Design review of the part built by this model. Coordinates are the model's own, in mm. Face numbers are marked on the shaded views. A direction names the side the tool comes from. Give positions to 0.01 mm unless a question says otherwise; leave off trailing zeros. Order: outer loops, then holes, each group sorted by start corner. A loop starts at its lowest first (then second) coordinate and runs counter-clockwise, first axis right, second up. Notation, with made-up numbers: (83, -39) -> (110, -39) arc R23 ccw to (110, -27) -> close; hole circle Ø9 at (43.25, 81). An arc over 180 degrees is marked (long way). Return JSON: item names as keys, results as strings.
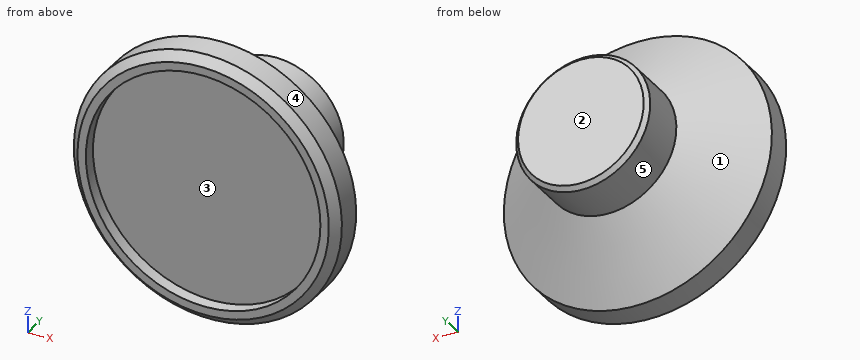
```python
from build123d import *

# Parameters (mm, degrees)
F2_SIZE  = 0.79375
F3_SIZE  = 1.5875
F4_R     = 22.225
F5_DEPTH = 2.3622


with BuildPart() as f1:
    # F0 (on Right) → F1 (revolve)
    with BuildSketch(Plane.YZ):
        Polygon((0, 25.4), (0, 0), (25.4, 0), (25.4, 12.7), (15.875, 12.7), (6.35, 25.4), align=None)
    revolve(axis=Axis((0, 12.7, 0), (0, -1, 0)))

    # F2
    f2_edges = [f1.edges().sort_by_distance(p)[0] for p in [
        (0, 25.4, -12.7),
    ]]
    chamfer(f2_edges, length=F2_SIZE)

    # F3
    f3_edges = [f1.edges().sort_by_distance(p)[0] for p in [
        (0, 0, -25.4),
    ]]
    chamfer(f3_edges, length=F3_SIZE)

    # F4 (on face) → F5 (cut)
    with BuildSketch(Plane.XZ):
        Circle(F4_R)
    extrude(amount=-F5_DEPTH, mode=Mode.SUBTRACT)


solid = f1.part
```
Item 1: Machinability: for the marked faces 4 and 5, which of the approach directions +Z, -Z, +X, -X, +Y, -Y give a long, thin tool a straight path to every point of the face, cutting with its end or side? Answer none if there is none.
Result set:
{"face 4": "+Y, -Y", "face 5": "+Y"}
Item 2: Wall thickness on L1, parallel to Z at x = 0, y = 0.5 (1 decimal); L2, parallel to Z at x = 0, y = 0.65 (1 decimal); L3, parallel to Y at x = -6.5, z = -8: over which ranges is each line inside the solid? List them lowest first. Write a range as [from, to].
Result set:
{"L1": "z = [-24.3, -22.2], [22.2, 24.3]", "L2": "z = [-24.5, -22.2], [22.2, 24.5]", "L3": "y = [2.36, 25.4]"}
Item 3: Add section C-C (y = 11.25). Give the boundary of the cut face in (x, z).
Result set:
{"outline": "circle Ø37.73 at (0, 0)"}
Item 4: Mouldability with a two-part tool opening along Z and no side actions: class the marked faces 1, 2 and 3 as released by +Z, released by -Z, zero draft, split by the parting line, or undercut.
Result set:
{"face 1": "split by the parting line", "face 2": "zero draft", "face 3": "undercut"}
Item 5: For pin 1 (3 mm diameter, centred on x = -12.5, z = -20, fed in from +Y); pin 2 (4 mm diameter, centred on x = -7, z = -13, fed in from -Y); pin 3 (6 mm diameter, centred on x = -18, y = 4.5, fed in from +Z), all flat-tipped, find the tip position at first contact; note any pin that passes through.
Result set:
{"pin 1": "stops at y = 8.84", "pin 2": "stops at y = 2.36", "pin 3": "stops at z = 20.5"}
